Geometry: final body of the model. Coordinates: model frame, mm. Face numbers are marked on the shaded views. A direction names the side the tool comes from. Round coordinates to 2 decimals unless told otherwise and drop trailing zeros. Write each loop counter-clockwise with the first axis right and the second up, starting at its lowest first coordinate (ties: lowest second). Pieces come first, ordered by that corner, then holes.
from build123d import *

# Parameters (mm, degrees)
CROQUIS1_W                       = 68
CROQUIS1_H                       = 46
BRIDA_BASE1_DEPTH                = 2
BRIDA_DE_ARISTA1_STRIP_W         = 9.4732
BRIDA_DE_ARISTA1_STRIP_H         = 2
BRIDA_DE_ARISTA1_STRIP_CUT_DEPTH = 46
BRIDA_DE_ARISTA1_DEPTH           = 46
BRIDA_DE_ARISTA2_STRIP_W         = 9.4732
BRIDA_DE_ARISTA2_STRIP_H         = 2
BRIDA_DE_ARISTA2_STRIP_CUT_DEPTH = 46
BRIDA_DE_ARISTA2_DEPTH           = 46
DESDOBLAR1_START                 = -131.122521377
DESDOBLAR1_DEPTH                 = 46
DESDOBLAR1_2_DEPTH               = 46
CROQUIS12_W                      = 137.245889802
CROQUIS12_H                      = 38
CORTAR_EXTRUIR1_DEPTH            = 2
DOBLAR1_START                    = -93.122521377
DOBLAR1_DEPTH                    = 8
DOBLAR1_2_DEPTH                  = 8


# Read off the part's stored shape, not the designer's step: Desdoblar1, Doblar1
# Sheet-metal steps are written as plain solids
with BuildPart() as part:
    # Croquis1 → Brida base1 (new body)
    with BuildSketch(Plane.XY.offset(452.5)):
        with Locations((-159.50357094, -108.122521377)):
            Rectangle(CROQUIS1_W, CROQUIS1_H)
    extrude(amount=-BRIDA_BASE1_DEPTH)

    # Brida de arista1 strip (across the edge) → Brida de arista1 strip cut (cut)
    with BuildSketch(Plane(origin=(-193.50357094, -131.122521377, 450.5), x_dir=(1, 0, 0), z_dir=(0, 1, 0))):
        with Locations((-2, -1)):
            Rectangle(BRIDA_DE_ARISTA1_STRIP_W, BRIDA_DE_ARISTA1_STRIP_H)
    extrude(amount=BRIDA_DE_ARISTA1_STRIP_CUT_DEPTH, mode=Mode.SUBTRACT)

    # Brida de arista1 section (across the edge) → Brida de arista1 (add)
    with BuildSketch(Plane(origin=(-193.50357094, -131.122521377, 450.5), x_dir=(1, 0, 0), z_dir=(0, 1, 0))):
        with BuildLine():
            Line((0, 0.7366), (0, 58))
            Line((0, 58), (2, 58))
            Line((2, 58), (2, 0.7366))
            ThreePointArc((2, 0.7366), (2.215745145, 0.215745145), (2.7366, 0))
            Line((2.7366, 0), (2.7366, -2))
            ThreePointArc((2.7366, -2), (0.801531583, -1.198468417), (0, 0.7366))
        make_face()
    extrude(amount=BRIDA_DE_ARISTA1_DEPTH)

    # Brida de arista2 strip (across the edge) → Brida de arista2 strip cut (cut)
    with BuildSketch(Plane(origin=(-193.50357094, -85.122521377, 392.5), x_dir=(0, 0, 1), z_dir=(0, -1, 0))):
        with Locations((-2, -1)):
            Rectangle(BRIDA_DE_ARISTA2_STRIP_W, BRIDA_DE_ARISTA2_STRIP_H)
    extrude(amount=BRIDA_DE_ARISTA2_STRIP_CUT_DEPTH, mode=Mode.SUBTRACT)

    # Brida de arista2 section (across the edge) → Brida de arista2 (add)
    with BuildSketch(Plane(origin=(-193.50357094, -85.122521377, 392.5), x_dir=(0, 0, 1), z_dir=(0, -1, 0))):
        with BuildLine():
            Line((0, 0.7366), (0, 78))
            Line((0, 78), (2, 78))
            Line((2, 78), (2, 0.7366))
            ThreePointArc((2, 0.7366), (2.215745145, 0.215745145), (2.7366, 0))
            Line((2.7366, 0), (2.7366, -2))
            ThreePointArc((2.7366, -2), (0.801531583, -1.198468417), (0, 0.7366))
        make_face()
    extrude(amount=BRIDA_DE_ARISTA2_DEPTH)

    # Desdoblar1 outline → Desdoblar1 (cut)
    with BuildSketch(Plane(origin=(0, 0, 0), x_dir=(1, 0, 0), z_dir=(0, 1, 0)).offset(DESDOBLAR1_START)):
        with BuildLine():
            ThreePointArc((-193.50357094, -449.7634), (-193.478203969, -450.135145906), (-193.402573338, -450.5))
            Line((-193.402573338, -450.5), (-190.76697094, -450.5))
            ThreePointArc((-190.76697094, -450.5), (-191.287825795, -450.284254855), (-191.50357094, -449.7634))
            Line((-191.50357094, -449.7634), (-191.50357094, -395.2366))
            ThreePointArc((-191.50357094, -395.2366), (-192.305102522, -393.301531582), (-194.24017094, -392.5))
            Line((-194.24017094, -392.5), (-271.50357094, -392.5))
            Line((-271.50357094, -392.5), (-271.50357094, -394.5))
            Line((-271.50357094, -394.5), (-194.24017094, -394.5))
            ThreePointArc((-194.24017094, -394.5), (-193.719316085, -394.715745145), (-193.50357094, -395.2366))
            Line((-193.50357094, -395.2366), (-193.50357094, -449.7634))
        make_face()
    extrude(amount=DESDOBLAR1_DEPTH, mode=Mode.SUBTRACT)

    # Desdoblar1 2 outline → Desdoblar1 2 (add)
    with BuildSketch(Plane(origin=(0, 0, 0), x_dir=(1, 0, 0), z_dir=(0, 1, 0)).offset(DESDOBLAR1_START)):
        with BuildLine():
            Line((-328.012860742, -452.5), (-190.76697094, -452.5))
            ThreePointArc((-190.76697094, -452.5), (-192.421238149, -451.943395312), (-193.402573338, -450.5))
            Line((-193.402573338, -450.5), (-328.012860742, -450.5))
            Line((-328.012860742, -450.5), (-328.012860742, -452.5))
        make_face()
    extrude(amount=DESDOBLAR1_2_DEPTH)

    # Croquis12 → Cortar-Extruir1 (cut)
    with BuildSketch(Plane.XY.offset(452.5)):
        with Locations((-259.389915841, -112.122521377)):
            Rectangle(CROQUIS12_W, CROQUIS12_H)
    extrude(amount=-CORTAR_EXTRUIR1_DEPTH, mode=Mode.SUBTRACT)

    # Doblar1 outline → Doblar1 (cut)
    with BuildSketch(Plane(origin=(0, 0, 0), x_dir=(1, 0, 0), z_dir=(0, 1, 0)).offset(DOBLAR1_START)):
        with BuildLine():
            ThreePointArc((-190.76697094, -452.5), (-192.421238149, -451.943395312), (-193.402573338, -450.5))
            Line((-193.402573338, -450.5), (-328.012860742, -450.5))
            Line((-328.012860742, -450.5), (-328.012860742, -452.5))
            Line((-328.012860742, -452.5), (-190.76697094, -452.5))
        make_face()
    extrude(amount=DOBLAR1_DEPTH, mode=Mode.SUBTRACT)

    # Doblar1 2 outline → Doblar1 2 (add)
    with BuildSketch(Plane(origin=(0, 0, 0), x_dir=(1, 0, 0), z_dir=(0, 1, 0)).offset(DOBLAR1_START)):
        with BuildLine():
            Line((-193.50357094, -395.2366), (-193.50357094, -449.7634))
            ThreePointArc((-193.50357094, -449.7634), (-193.478203969, -450.135145906), (-193.402573338, -450.5))
            Line((-193.402573338, -450.5), (-190.76697094, -450.5))
            ThreePointArc((-190.76697094, -450.5), (-191.287825795, -450.284254855), (-191.50357094, -449.7634))
            Line((-191.50357094, -449.7634), (-191.50357094, -395.2366))
            ThreePointArc((-191.50357094, -395.2366), (-192.305102522, -393.301531582), (-194.24017094, -392.5))
            Line((-194.24017094, -392.5), (-271.50357094, -392.5))
            Line((-271.50357094, -392.5), (-271.50357094, -394.5))
            Line((-271.50357094, -394.5), (-194.24017094, -394.5))
            ThreePointArc((-194.24017094, -394.5), (-193.719316085, -394.715745145), (-193.50357094, -395.2366))
        make_face()
    extrude(amount=DOBLAR1_2_DEPTH)


solid = part.part
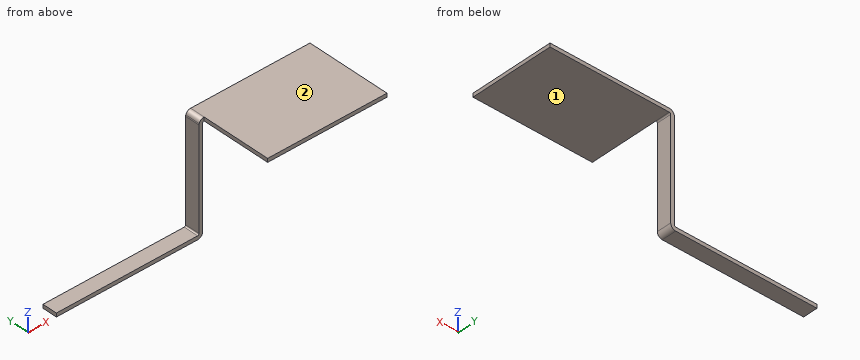
1) Section A-A on y = -90.5. Output: boundary loops of the cut face in (x, z).
2) Section B-B on x = -240. Output: boundary loops of the cut face in (y, z), plus the area to 3 significant figures.
3) Section C-C on z = 404.5. Output: boundary loops of the cut face in (x, y).
4) First-contact query: P1, Ø9, axis at y = -89, z = 432.5, coming from the -X side; P2, Ø6.5, axis at x = -243, y = -89.5, coming from the +Z side; P3, Ø2, axis at y = -115.5, z = 451.5, coming from the -X side. Flat tips, straight axial feed; report the tip coordinate or a pass-through.
5) Reachability of the marked faces 1 and 2 from +Z, -Z, +X, -X, +Y, -Y: full face, straight path, thin tool, end or side. Return the list, or none.
6) Line query: probe 1 along Z at (x, y) = (-152, -111.5); probe 2 along Z at (x, y) = (-216, -92). Output: solid intervals per line, ascending.
Filled in:
1. outline: (-271.5, 392.5) - (-194.24, 392.5) arc R2.74 ccw to (-191.5, 395.24) - (-191.5, 449.76) arc R0.74 cw to (-190.77, 450.5) - (-125.5, 450.5) - (-125.5, 452.5) - (-190.77, 452.5) arc R2.74 ccw to (-193.5, 449.76) - (-193.5, 395.24) arc R0.74 cw to (-194.24, 394.5) - (-271.5, 394.5) - close
2. outline: (-93.12, 392.5) - (-85.12, 392.5) - (-85.12, 394.5) - (-93.12, 394.5) - close
2. area: 16.0 mm2
3. outline: (-193.5, -93.12) - (-191.5, -93.12) - (-191.5, -85.12) - (-193.5, -85.12) - close
4. P1: stops at x = -193.5
4. P2: stops at z = 394.5
4. P3: stops at x = -190.77
5. face 1: -Z, +X, +Y, -Y
5. face 2: +Z, +X, -X, +Y, -Y
6. probe 1: z = 450.5 to 452.5
6. probe 2: z = 392.5 to 394.5
